For this review, take the finished solid that the model builds, in its own axes (mm). A direction names the side the tool comes from. Coordinates: 2 decimals unless noted, no trailing zeros. Order: outer loops, then holes, each group sorted by start corner. A loop starts at its lowest first (then second) coordinate and runs counter-clockwise, first axis right, second up. Notation, with made-up numbers: M 69.5,-14 L 92.5,-14 A8 ccw 92.5,-4 Z; hole C -18,33.25 d10. An arc over 180 degrees is marked long. Use one line per item in the form item = value. Start each with the question number.
```python
from build123d import *

# Parameters (mm, degrees)
F0_W     = 645
F0_H     = 430
F1_DEPTH = 15
F3_D     = 13.2
F4_R     = 8.5
F5_DEPTH = 15


with BuildPart() as f1:
    # F0 (on Top) → F1 (new body)
    with BuildSketch(Plane.XY):
        Rectangle(F0_W, F0_H)
        Polygon((-132.5, 120), (-117.5, 135), (207.5, 135), (222.5, 120), (222.5, -120), (207.5, -135), (-117.5, -135), (-132.5, -120), align=None, mode=Mode.SUBTRACT)
    extrude(amount=F1_DEPTH)

    # F3 (through all)
    with Locations(Plane(origin=(0, 0, 0), x_dir=(1, 0, 0), z_dir=(0, 0, -1))):
        with Locations((-297.5, -150), (-297.5, 0), (-297.5, 150), (-157.5, -150), (-157.5, 0), (-157.5, 150), (-32.5, 185), (57.5, 185), (212.5, 185), (302.5, 185), (302.5, -185), (212.5, -185), (57.5, -185), (-32.5, -185)):
            Hole(F3_D / 2)

    # F4 (on Top) → F5 (cut, through all)
    with BuildSketch(Plane.XY):
        with Locations((-87.5, 185)):
            Circle(F4_R)
        with Locations((162.5, 185)):
            Circle(F4_R)
        with Locations((162.5, -185)):
            Circle(F4_R)
        with Locations((-87.5, -185)):
            Circle(F4_R)
    extrude(amount=F5_DEPTH, mode=Mode.SUBTRACT)


solid = f1.part
```
1. Consider section B-B, the plane z = 2.5. Give the number of separate pieces and of enclosed holes in the cut face, plus the area to 3 significant figures.
2. Consider section D-D, the plane x = 302.5. Write out the cut boundary in (y, z).
3. Tool access review of faces 4 (the flat face through (47, -135, 7)), 5 (the flat face through (-322.5, -3, 7)): name each direction out of +Z, -Z, +X, -X, +Y, -Y from which nothing blocks a thin tool from reaching the whole face with its end or side.
4. To check wall thickness, follow line 1 (Y direction, x = -32, z = 14.25); line 2 (Y direction, x = -297.5, z = 6.5); line 3 (X direction, y = -99.5, z = 2). State the ranges of each line that lie inside material, in increasing order.
5. The part is to be moulded in two halves that separate along Y. For faces 1 (the flat face through (-5, -215, 7)), 2 (the flat face through (222.5, 2, 7)), 3 (the flat face through (322.5, -3, 7)), say which applies: pulls with the +Y half, pulls with the -Y half, needs draft (parallel to the pull), parting line crosses it, or undercut.
6. Consider section A-A, the plane x = -157.5. Write out the cut boundary in (y, z), plus the area to 3 significant figures.
7. Consider section C-C, the plane y = 74. Write out the cut boundary in (x, z), plus the area to 3 significant figures.
Answers follow:
q1.separate_pieces = 1
q1.enclosed_holes = 19
q1.area = 179,000 mm²
q2.outline = M -215,0 L -191.6,0 L -191.6,15 L -215,15 Z; M -178.4,0 L 178.4,0 L 178.4,15 L -178.4,15 Z; M 191.6,0 L 215,0 L 215,15 L 191.6,15 Z
q3.face_4 = +Z, -Z
q3.face_5 = +Z, -Z, -X, +Y, -Y
q4.line_1 = -215 to -191.58, -178.42 to -135, 135 to 178.42, 191.58 to 215
q4.line_2 = -215 to -156.6, -143.4 to -6.6, 6.6 to 143.4, 156.6 to 215
q4.line_3 = -322.5 to -132.5, 222.5 to 322.5
q5.face_1 = pulls with the -Y half
q5.face_2 = undercut
q5.face_3 = needs draft
q6.outline = M -215,0 L -156.6,0 L -156.6,15 L -215,15 Z; M -143.4,0 L -6.6,0 L -6.6,15 L -143.4,15 Z; M 6.6,0 L 143.4,0 L 143.4,15 L 6.6,15 Z; M 156.6,0 L 215,0 L 215,15 L 156.6,15 Z
q6.area = 5,860 mm²
q7.outline = M -322.5,0 L -132.5,0 L -132.5,15 L -322.5,15 Z; M 222.5,0 L 322.5,0 L 322.5,15 L 222.5,15 Z
q7.area = 4,350 mm²
